The listing builds one solid part. Answer for the finished solid, in the listing's coordinates (mm). Give positions to 0.01 mm unless a question says otherwise; leave off trailing zeros. Order: outer loops, then holes, each group sorted by start corner. A loop starts at its lowest first (then second) coordinate and runs counter-clockwise, first axis right, second up. Notation, with made-up numbers: (25.25, 10) - (42.25, 10) arc R7 cw to (42.25, 19) - close; hole circle Ø3 at (31, 54). An arc over 180 degrees is marked (long way). Answer in a Markdown table with one row per item.
from build123d import *

# Parameters (mm, degrees)
F1_DEPTH     = 25.4
F2_R         = 24.2182856507
F3_DEPTH     = 25.401
F5_T1_DEPTH  = 114.3
F5_T3_DEPTH  = 241.3
F5_T6_ANGLE  = 90
F5_T8_ANGLE  = 90
F5_T10_ANGLE = 90
F5_T12_ANGLE = 90
F5_T14_ANGLE = 90
F5_T16_ANGLE = 90
F5_T18_ANGLE = 90
F5_T20_ANGLE = 90


# Not quite as in the source:
# - a fillet or chamfer that OpenCascade refuses, or shapes differently, is made with other operations: its cross-section is extruded or revolved along the edge and cut away or added
# - a feature of the source that left no trace in its solid (it failed there, or was rolled back) is left out


with BuildPart() as f1:
    # F0 (on Top) → F1 (new body)
    with BuildSketch(Plane.XY):
        with BuildLine():
            Line((120.65, 63.5), (-120.65, 63.5))
            ThreePointArc((-120.65, 63.5), (-125.1401280605, 61.6401280605), (-127, 57.15))
            Line((-127, 57.15), (-127, -57.15))
            ThreePointArc((-127, -57.15), (-125.1401280605, -61.6401280605), (-120.65, -63.5))
            Line((-120.65, -63.5), (120.65, -63.5))
            ThreePointArc((120.65, -63.5), (125.1401280605, -61.6401280605), (127, -57.15))
            Line((127, -57.15), (127, 57.15))
            ThreePointArc((127, 57.15), (125.1401280605, 61.6401280605), (120.65, 63.5))
        make_face()
    extrude(amount=F1_DEPTH)

    # F2 (on face) → F3 (cut, through all)
    with BuildSketch(Plane.XY.offset(25.4)):
        with Locations((-101.6, 12.7)):
            Circle(F2_R)
    extrude(amount=-F3_DEPTH, mode=Mode.SUBTRACT)

    # F5: fillet of radius 5.08 on 16 edges, made by hand

    # F5_s2 → F5_t1 (cut)
    with BuildSketch(Plane.XZ.offset(-57.15)):
        with BuildLine():
            ThreePointArc((121.92, 0), (125.5121024484, 1.4878975516), (127, 5.08))
            Line((127, 5.08), (127, 0))
            Line((127, 0), (121.92, 0))
        make_face()
        with BuildLine():
            ThreePointArc((-121.92, 0), (-125.5121024484, 1.4878975516), (-127, 5.08))
            Line((-127, 5.08), (-127, 0))
            Line((-127, 0), (-121.92, 0))
        make_face()
        with BuildLine():
            ThreePointArc((121.92, 25.4), (125.5121024484, 23.9121024484), (127, 20.32))
            Line((127, 20.32), (127, 25.4))
            Line((127, 25.4), (121.92, 25.4))
        make_face()
        with BuildLine():
            ThreePointArc((-121.92, 25.4), (-125.5121024484, 23.9121024484), (-127, 20.32))
            Line((-127, 20.32), (-127, 25.4))
            Line((-127, 25.4), (-121.92, 25.4))
        make_face()
    extrude(amount=F5_T1_DEPTH, mode=Mode.SUBTRACT)

    # F5_s4 → F5_t3 (cut)
    with BuildSketch(Plane.YZ.offset(-120.65)):
        with BuildLine():
            ThreePointArc((63.5, 5.08), (62.0121024484, 1.4878975516), (58.42, 0))
            Line((58.42, 0), (63.5, 0))
            Line((63.5, 0), (63.5, 5.08))
        make_face()
        with BuildLine():
            ThreePointArc((63.5, 20.32), (62.0121024484, 23.9121024484), (58.42, 25.4))
            Line((58.42, 25.4), (63.5, 25.4))
            Line((63.5, 25.4), (63.5, 20.32))
        make_face()
        with BuildLine():
            ThreePointArc((-58.42, 0), (-62.0121024484, 1.4878975516), (-63.5, 5.08))
            Line((-63.5, 5.08), (-63.5, 0))
            Line((-63.5, 0), (-58.42, 0))
        make_face()
        with BuildLine():
            ThreePointArc((-58.42, 25.4), (-62.0121024484, 23.9121024484), (-63.5, 20.32))
            Line((-63.5, 20.32), (-63.5, 25.4))
            Line((-63.5, 25.4), (-58.42, 25.4))
        make_face()
    extrude(amount=F5_T3_DEPTH, mode=Mode.SUBTRACT)

    # F5_s5 → F5_t6 (revolve, cut)
    with BuildSketch(Plane.XZ.offset(-57.15)):
        with BuildLine():
            ThreePointArc((127, 5.08), (125.5121024484, 1.4878975516), (121.92, 0))
            Line((121.92, 0), (127, 0))
            Line((127, 0), (127, 5.08))
        make_face()
    revolve(axis=Axis((120.65, 57.15, 0), (0, 0, 1)), revolution_arc=F5_T6_ANGLE, mode=Mode.SUBTRACT)

    # F5_s7 → F5_t8 (revolve, cut)
    with BuildSketch(Plane.XZ.offset(-57.15)):
        with BuildLine():
            ThreePointArc((127, 20.32), (125.5121024484, 23.9121024484), (121.92, 25.4))
            Line((121.92, 25.4), (127, 25.4))
            Line((127, 25.4), (127, 20.32))
        make_face()
    revolve(axis=Axis((120.65, 57.15, 25.4), (0, 0, 1)), revolution_arc=F5_T8_ANGLE, mode=Mode.SUBTRACT)

    # F5_s9 → F5_t10 (revolve, cut)
    with BuildSketch(Plane.YZ.offset(-120.65)):
        with BuildLine():
            ThreePointArc((63.5, 5.08), (62.0121024484, 1.4878975516), (58.42, 0))
            Line((58.42, 0), (63.5, 0))
            Line((63.5, 0), (63.5, 5.08))
        make_face()
    revolve(axis=Axis((-120.65, 57.15, 0), (0, 0, 1)), revolution_arc=F5_T10_ANGLE, mode=Mode.SUBTRACT)

    # F5_s11 → F5_t12 (revolve, cut)
    with BuildSketch(Plane.YZ.offset(-120.65)):
        with BuildLine():
            ThreePointArc((63.5, 20.32), (62.0121024484, 23.9121024484), (58.42, 25.4))
            Line((58.42, 25.4), (63.5, 25.4))
            Line((63.5, 25.4), (63.5, 20.32))
        make_face()
    revolve(axis=Axis((-120.65, 57.15, 25.4), (0, 0, 1)), revolution_arc=F5_T12_ANGLE, mode=Mode.SUBTRACT)

    # F5_s13 → F5_t14 (revolve, cut)
    with BuildSketch(Plane.YZ.offset(120.65)):
        with BuildLine():
            ThreePointArc((-58.42, 0), (-62.0121024484, 1.4878975516), (-63.5, 5.08))
            Line((-63.5, 5.08), (-63.5, 0))
            Line((-63.5, 0), (-58.42, 0))
        make_face()
    revolve(axis=Axis((120.65, -57.15, 0), (0, 0, 1)), revolution_arc=F5_T14_ANGLE, mode=Mode.SUBTRACT)

    # F5_s15 → F5_t16 (revolve, cut)
    with BuildSketch(Plane.XZ.offset(57.15)):
        with BuildLine():
            ThreePointArc((-121.92, 0), (-125.5121024484, 1.4878975516), (-127, 5.08))
            Line((-127, 5.08), (-127, 0))
            Line((-127, 0), (-121.92, 0))
        make_face()
    revolve(axis=Axis((-120.65, -57.15, 0), (0, 0, 1)), revolution_arc=F5_T16_ANGLE, mode=Mode.SUBTRACT)

    # F5_s17 → F5_t18 (revolve, cut)
    with BuildSketch(Plane.YZ.offset(120.65)):
        with BuildLine():
            ThreePointArc((-58.42, 25.4), (-62.0121024484, 23.9121024484), (-63.5, 20.32))
            Line((-63.5, 20.32), (-63.5, 25.4))
            Line((-63.5, 25.4), (-58.42, 25.4))
        make_face()
    revolve(axis=Axis((120.65, -57.15, 25.4), (0, 0, 1)), revolution_arc=F5_T18_ANGLE, mode=Mode.SUBTRACT)

    # F5_s19 → F5_t20 (revolve, cut)
    with BuildSketch(Plane.XZ.offset(57.15)):
        with BuildLine():
            ThreePointArc((-121.92, 25.4), (-125.5121024484, 23.9121024484), (-127, 20.32))
            Line((-127, 20.32), (-127, 25.4))
            Line((-127, 25.4), (-121.92, 25.4))
        make_face()
    revolve(axis=Axis((-120.65, -57.15, 25.4), (0, 0, 1)), revolution_arc=F5_T20_ANGLE, mode=Mode.SUBTRACT)


solid = f1.part
Item 1: Consider line 1 (Y direction, x = -101.6, z = 11.75); line 2 (X direction, y = 12.7, z = 5.75); line 3 (X direction, y = 5, z = 24.5). Determine where each line is inside the solid, lowest interval first.
Answer block:
| item | result |
|---|---|
| line 1 | -63.5 to -11.52, 36.92 to 63.5 |
| line 2 | -127 to -125.82, -77.38 to 127 |
| line 3 | -124.81 to -124.56, -78.64 to 124.81 |
Item 2: Each of these flat-tipped pins is pushed along its axis until it touches: P1, Ø1, axis at y = 44.5, z = 21.5, coming from the +X side; P2, Ø12, axis at x = 84, z = 20.5, coming from the +Y side. Where does it stop, or does it pass through?
Answer block:
| item | result |
|---|---|
| P1 | x = 126.95 |
| P2 | y = 63.5 |
Item 3: Find section D-D on y = -8. Write down the section's boundary in (x, z), then the cut area to 3 significant figures.
Answer block:
| item | result |
|---|---|
| outline | (-127, 5.08) arc R5.08 ccw to (-121.92, 0) - (-114.17, 0) - (-114.17, 25.4) - (-121.92, 25.4) arc R5.08 ccw to (-127, 20.32) - close; (-89.03, 0) - (121.92, 0) arc R5.08 ccw to (127, 5.08) - (127, 20.32) arc R5.08 ccw to (121.92, 25.4) - (-89.03, 25.4) - close |
| area | 5,790 mm² |
Item 4: Find section A-A on x = -101.6. Write down the section's boundary in (y, z), then the cut area to 3 significant figures.
Answer block:
| item | result |
|---|---|
| outline | (-63.5, 5.08) arc R5.08 ccw to (-58.42, 0) - (-11.52, 0) - (-11.52, 25.4) - (-58.42, 25.4) arc R5.08 ccw to (-63.5, 20.32) - close; (36.92, 0) - (58.42, 0) arc R5.08 ccw to (63.5, 5.08) - (63.5, 20.32) arc R5.08 ccw to (58.42, 25.4) - (36.92, 25.4) - close |
| area | 1,970 mm² |
Item 5: Find section C-C on y = 15. Write down the section's boundary in (x, z), then the cut area to 3 significant figures.
Answer block:
| item | result |
|---|---|
| outline | (-127, 5.08) arc R5.08 ccw to (-125.71, 1.7) - (-125.71, 23.7) arc R5.08 ccw to (-127, 20.32) - close; (-77.49, 0) - (121.92, 0) arc R5.08 ccw to (127, 5.08) - (127, 20.32) arc R5.08 ccw to (121.92, 25.4) - (-77.49, 25.4) - close |
| area | 5,210 mm² |
Item 6: Find section B-B on z = 15. Write down the section's boundary in (x, y).
Answer block:
| item | result |
|---|---|
| outline | (-127, -57.15) arc R6.35 ccw to (-120.65, -63.5) - (120.65, -63.5) arc R6.35 ccw to (127, -57.15) - (127, 57.15) arc R6.35 ccw to (120.65, 63.5) - (-120.65, 63.5) arc R6.35 ccw to (-127, 57.15) - close; hole circle Ø48.44 at (-101.6, 12.7) |
